The listing builds one solid part. Answer for the finished solid, in the listing's coordinates (mm). A direction names the side the tool comes from. Round coordinates to 2 decimals unless told otherwise and drop trailing zeros. Loops run counter-clockwise (first coordinate to the right, second up) from the corner with the lowest first, then second, coordinate; pieces in that order, holes last. Notation, with made-up numbers: M 48.25,-17.75 L 85.25,-17.75 A22 cw 85.25,9.25 Z; hole C 71.5,22.25 d8. An arc over 180 degrees is marked long. Answer as a JSON object with one key per item and string values.
```python
from build123d import *

# Parameters (mm, degrees)
SKETCH_1_R          = 2.75
SKETCH_1_R_2        = 14
EXTRUDE_1_DEPTH     = 10
SKETCH_1_3_R        = 14
SKETCH_1_3_R_2      = 8
EXTRUDE_2_DEPTH     = 47
SKETCH_2_R          = 3
CUT_EXTRUDE_1_DEPTH = 20


with BuildPart() as part:
    # Sketch 1 → Extrude 1 (new body)
    with BuildSketch(Plane(origin=(0, 0, 0), x_dir=(1, 0, 0), z_dir=(0, 1, 0))):
        with BuildLine():
            Line((20, 13.266499161), (20, -13.266499161))
            ThreePointArc((20, -13.266499161), (0, -24), (-20, -13.266499161))
            Line((-20, -13.266499161), (-20, 13.266499161))
            ThreePointArc((-20, 13.266499161), (0, 24), (20, 13.266499161))
        make_face()
        with Locations((0, 19)):
            Circle(SKETCH_1_R, mode=Mode.SUBTRACT)
        with Locations((13.435028843, 13.435028843)):
            Circle(SKETCH_1_R, mode=Mode.SUBTRACT)
        Circle(SKETCH_1_R_2, mode=Mode.SUBTRACT)
        with Locations((0, -19)):
            Circle(SKETCH_1_R, mode=Mode.SUBTRACT)
        with Locations((-13.435028843, -13.435028843)):
            Circle(SKETCH_1_R, mode=Mode.SUBTRACT)
        with Locations((13.435028843, -13.435028843)):
            Circle(SKETCH_1_R, mode=Mode.SUBTRACT)
        with Locations((-13.435028843, 13.435028843)):
            Circle(SKETCH_1_R, mode=Mode.SUBTRACT)
    extrude(amount=EXTRUDE_1_DEPTH)

    # Sketch 1_3 → Extrude 2 (add)
    with BuildSketch(Plane(origin=(0, 0, 0), x_dir=(1, 0, 0), z_dir=(0, 1, 0))):
        Circle(SKETCH_1_3_R)
        Circle(SKETCH_1_3_R_2, mode=Mode.SUBTRACT)
    extrude(amount=EXTRUDE_2_DEPTH)

    # Sketch 2 → Cut-Extrude 1 (cut)
    with BuildSketch(Plane.ZY.offset(20)):
        with Locations((0, 5)):
            Circle(SKETCH_2_R)
    extrude(amount=-CUT_EXTRUDE_1_DEPTH, mode=Mode.SUBTRACT)


solid = part.part
```
Item 1: The part is cut by section A-A (x = 0). Give the vertices of the cut face in (y, z).
Values follow:
{"outline": "M 0,-24 L 10,-24 L 10,-21.75 L 0,-21.75 Z; M 0,-16.25 L 10,-16.25 L 10,-14 L 47,-14 L 47,-8 L 0,-8 Z; M 0,8 L 47,8 L 47,14 L 10,14 L 10,16.25 L 0,16.25 Z; M 0,21.75 L 10,21.75 L 10,24 L 0,24 Z"}
Item 2: Flat-ended cylindrical pins translate along their axes: P1, Ø10, axis at x = -0.5, y = 40, coming from the +Z side; P2, Ø3.5, axis at x = 0, z = 19, coming from the +Y side; P3, Ø6.5, axis at x = -13.44, z = -13.44, coming from the +Y side; P4, Ø8, axis at x = -15.5, y = 26.5, coming from the -Z side. Find the tip coordinate at first contact, or state that the pin passes through.
Values follow:
{"P1": "z = 14", "P2": "through", "P3": "y = 10", "P4": "z = -7.98"}
Item 3: The part is cut by section D-D (y = 3). Give the vertices of the cut face in (x, z).
Values follow:
{"outline": "M -20,-13.27 A24 ccw 20,-13.27 L 20,13.27 A24 ccw -20,13.27 L -20,2.24 L -7.68,2.24 A8 cw long -7.68,-2.24 L -20,-2.24 Z; hole C -13.44,-13.44 d5.5; hole C -13.44,13.44 d5.5; hole C 0,-19 d5.5; hole C 0,19 d5.5; hole C 13.44,-13.44 d5.5; hole C 13.44,13.44 d5.5"}
Item 4: The part is cut by section C-C (z = 7). Give the vertices of the cut face in (x, y).
Values follow:
{"outline": "M -20,0 L -3.87,0 L -3.87,47 L -12.12,47 L -12.12,10 L -20,10 Z; M 3.87,0 L 20,0 L 20,10 L 12.12,10 L 12.12,47 L 3.87,47 Z"}
Item 5: Which of the six approach directions +Z, -Z, +X, -X, +Y, -Y give full straight-line access (tool end or side, diameter ignored) to faces 1 (the face through (-13.8, 2.07, -0.65)), 2 (the face through (-0.358, 4.93, -21.727)), 3 (the face through (9, 10, -11))?
Values follow:
{"face 1": "-X", "face 2": "+Y, -Y", "face 3": "+Y"}
Item 6: The part is cut by section B-B (z = 0). Give the vertices of the cut face in (x, y).
Values follow:
{"outline": "M -20,0 L -8,0 L -8,2 L -20,2 Z; M -20,8 L -8,8 L -8,47 L -14,47 L -14,10 L -20,10 Z; M 8,0 L 20,0 L 20,10 L 14,10 L 14,47 L 8,47 Z"}
Item 7: Straight lines are drawn through the part: line 1 (Y direction, x = -12.5, z = 0); line 2 (Z direction, x = -0.5, y = 38); line 3 (Y direction, x = 17.5, z = -11). For each, find the intervals that lie inside material, in ascending order.
Values follow:
{"line 1": "0 to 2, 8 to 47", "line 2": "-13.99 to -7.98, 7.98 to 13.99", "line 3": "0 to 10"}
Item 8: Determine the mould class of faces 4 (the face through (11.408, 4.93, -15.294)), 5 (the face through (6, 47, 6)), 6 (the face through (10.688, 4.93, 13.314)), 7 (the face through (0, 5, 24)) for opening direction X: released by +X, released by -X, zero draft, split by the parting line, or undercut.
Values follow:
{"face 4": "undercut", "face 5": "zero draft", "face 6": "undercut", "face 7": "split by the parting line"}
